Autodesk Inventor part; units mm, degrees
ref_plane "YZ Plane" through (0, 0, 0) normal (1, 0, 0) x (0, 1, 0)
ref_plane "XZ Plane" through (0, 0, 0) normal (0, 1, 0) x (-1, 0, 0)
ref_plane "XY Plane" through (0, 0, 0) normal (0, 0, 1) x (1, 0, 0)
sketch "Sketch1" plane through (0, 0, 0) normal (0, 0, 1) x (1, 0, 0)
  line L0 (0, 0) -> (12.5, 0) construction
  line L1 (12.5, 0) -> (12.5, 17) construction
  line L2 (12.5, 17) -> (0, 17) construction
  line L3 (0, 17) -> (0, 0) construction
  line L4 (5, 3) -> (11, 3) construction
  line L5 (11, 3) -> (11, 15) construction
  line L6 (11, 15) -> (5, 15) construction
  line L7 (5, 15) -> (5, 3) construction
  line L8 (-10, 22) -> (22.5, 22)
  line L9 (22.5, 22) -> (22.5, -5)
  line L10 (22.5, -5) -> (-10, -5)
  line L11 (-10, -5) -> (-10, 22)
  circle A0 centre (-5.5, 18.5) radius 2.05
  circle A1 centre (-5.5, -1.5) radius 2.05
  circle A2 centre (18, -1.5) radius 2.05
  circle A3 centre (18, 18.5) radius 2.05
  point P0 (10, 14)
  dimension "d0" = 12.5
  dimension "d1" = 17
  dimension "d2" = 6
  dimension "d3" = 12
  dimension "d4" = 5
  dimension "d5" = 2
  dimension "d6" = 1
  dimension "d7" = 1
  dimension "d8" = 32.5
  dimension "d9" = 27
  dimension "d10" = 5
  dimension "d11" = 10
  dimension "d12" = 4.1
  dimension "d13" = 4.1
  dimension "d14" = 4.1
  dimension "d15" = 4.1
  dimension "d16" = 3.5
  dimension "d17" = 3.5
  dimension "d18" = 3.5
  dimension "d19" = 3.5
  dimension "d20" = 4.5
  dimension "d21" = 4.5
  dimension "d22" = 4.5
  dimension "d23" = 4.5
extrude "Extrusion1" add sketch "Sketch1" along normal blind 3
hole "Hole1" at (10, 14, 0) at (5, 15, 0) at (5, 3, 0) at (11, 3, 0) direction (0, 0, 1) diameter 2.1 end through all
fillet "Fillet1" radius 2 4 edges at (-10, 22, 1.5) (22.5, 22, 1.5) (22.5, -5, 1.5) (-10, -5, 1.5)
properties part number "Pump Mounting Plate"
Read the model definition and answer for the solid it produces. Units are mm, in the model's axes. Give positions to 0.01 mm unless a question says otherwise; leave off trailing zeros. Write each loop counter-clockwise with the first axis right and the second up, starting at its lowest first coordinate (ties: lowest second). Pieces come first, ordered by that corner, then holes. Notation, with made-up numbers: (37.5, 75.25) -> (96.5, 75.25) arc R20 ccw to (96.5, 93.25) -> close; hole circle Ø1 at (69, -4.5). An arc over 180 degrees is marked (long way). Answer as a JSON object with one key per item and string values. Group by question number.
1) Find section C-C (y = 3). Write down the section's boundary in (x, z), and give its area (3 significant figures).
2) Find section B-B (z = 0.85). Count the separate pieces of the cut face and the enclosed holes in it, and give its area (3 significant figures).
3) The mould has two halves that part along Y. Classify faces 1 (the flat face through (6, -5, 1)), 2 (the cylindrical face through (-7, 17.1, 1.5)), 3 (the flat face through (6, 9, 0)): +Y half, -Y half, draft (parallel to the pull), parting line (faces both ways), or undercut.
4) Consider L1, parallel to Y at x = 5, z = 0.1; L2, parallel to Y at x = 18, z = 1.95; L3, parallel to X at y = 3, z = 1.9. Determine where each line is inside the solid, lowest interval first. Write a range as from..to.
5) Find section A-A (x = -5.5). Write down the section's boundary in (y, z).
Values follow:
{
 "1": {"outline": "(-10, 0) -> (3.95, 0) -> (3.95, 3) -> (-10, 3) -> close; (6.05, 0) -> (9.95, 0) -> (9.95, 3) -> (6.05, 3) -> close; (12.05, 0) -> (22.5, 0) -> (22.5, 3) -> (12.05, 3) -> close", "area": "84.9 mm2"},
 "2": {"separate pieces": "1", "enclosed holes": "8", "area": "807 mm2"},
 "3": {"face 1": "-Y half", "face 2": "undercut", "face 3": "draft"},
 "4": {"L1": "y = -5..1.95, 4.05..13.95, 16.05..22", "L2": "y = -5..-3.55, 0.55..16.45, 20.55..22", "L3": "x = -10..3.95, 6.05..9.95, 12.05..22.5"},
 "5": {"outline": "(-5, 0) -> (-3.55, 0) -> (-3.55, 3) -> (-5, 3) -> close; (0.55, 0) -> (16.45, 0) -> (16.45, 3) -> (0.55, 3) -> close; (20.55, 0) -> (22, 0) -> (22, 3) -> (20.55, 3) -> close"}
}
